from build123d import *

# Parameters (mm, degrees)
BASE_FLANGE1_DEPTH = 10
FILLET_1_0_R       = 1


# Sheet-metal steps are written as plain solids
with BuildPart() as part:
    # Sketch1 → Base-Flange1 (new body)
    with BuildSketch(Plane(origin=(0, 0, 0), x_dir=(1, 0, 0), z_dir=(0, 1, 0))):
        Polygon((-400.811710089, 160), (400.811710089, 160), (412, 0), (-412, 0), align=None)
    extrude(amount=-BASE_FLANGE1_DEPTH)

    # Fillet-1.0
    fillet_1_0_edges = [part.edges().sort_by_distance(p)[0] for p in [
        (-400.811710089, -5, -160),
        (400.811710089, -5, -160),
        (412, -5, 0),
        (-412, -5, 0),
    ]]
    fillet(fillet_1_0_edges, radius=FILLET_1_0_R)


solid = part.part
The listing builds one solid part. Answer for the finished solid, in the listing's coordinates (mm). Round coordinates to 2 decimals unless told otherwise and drop trailing zeros. Write each loop counter-clockwise with the first axis right and the second up, starting at its lowest first coordinate (ties: lowest second). Pieces come first, ordered by that corner, then holes. Notation, with made-up numbers: (36, -34.75) - (74, -34.75) arc R4 ccw to (74, -30.75) - close; hole circle Ø2 at (18, 40.25). An arc over 180 degrees is marked (long way). Use one line per item in the form item = value. Start each with the question number.
Item 1: Find the intervals of material crossed by line 1 (X direction, y = -3.75, z = -10.5); line 2 (X direction, y = -6.5, z = -37), in increasing order. Write a range as [from, to].
Item 2: Flat-ended cylindrical pins translate along their axes: pin 1 Ø5 at (y, z) = (-6.5, -71.5) entering from -X; pin 2 Ø5 at (y, z) = (-8.5, -135.5) entering from -X; pin 3 Ø6 at (y, z) = (-2, -110.5) entering from -X. Find the tip coordinate at first contact, or state that the pin passes through.
Item 3: A cutting plane is placed at A-A (z = -125). Write down the section's boundary in (x, y).
The answers:
q1.line_1 = [-411.27, 411.27]
q1.line_2 = [-409.41, 409.41]
q2.pin_1 = -407.18
q2.pin_2 = -402.7
q2.pin_3 = -404.48
q3.outline = (-403.26, -10) - (403.26, -10) - (403.26, 0) - (-403.26, 0) - close
